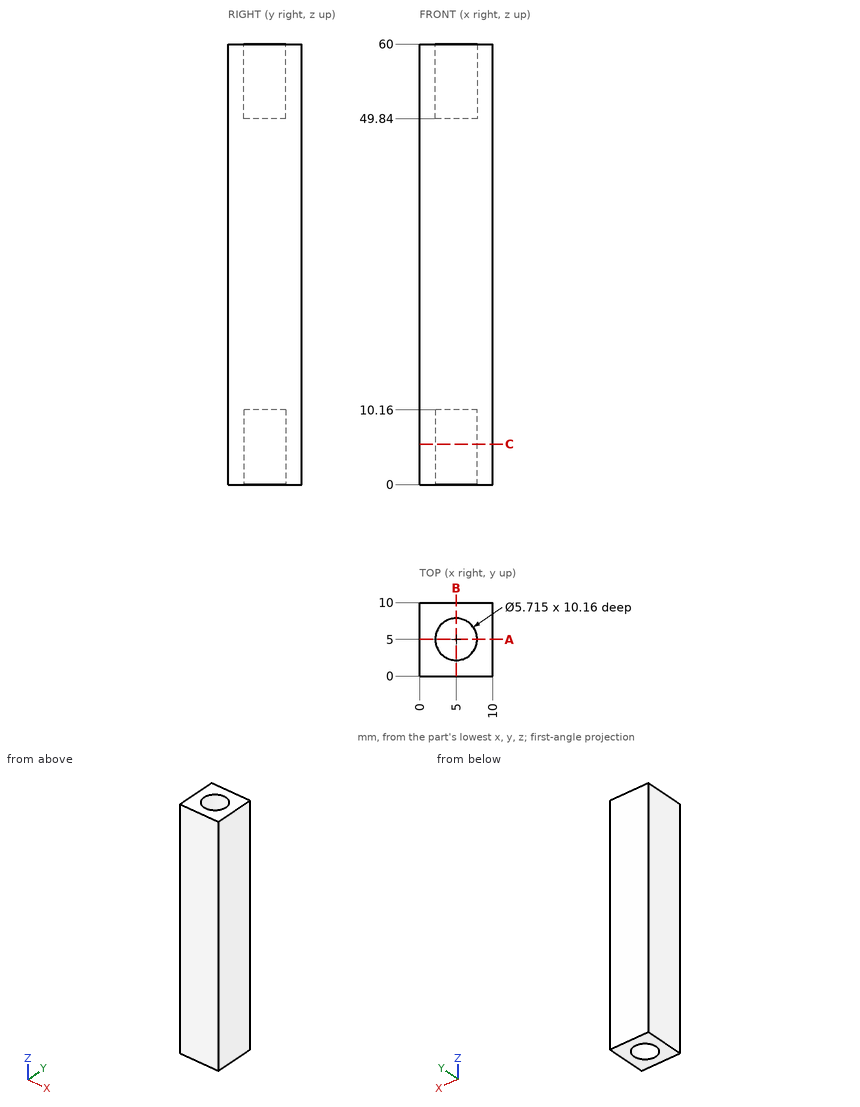
The drawing under review shows one solid part. Ordinate dimensions are in mm from its lowest x, y, z. Coordinates: 2 decimals unless noted, no trailing zeros. Order: outer loops, then holes, each group sorted by start corner. A loop starts at its lowest first (then second) coordinate and runs counter-clockwise, first axis right, second up. Notation, with made-up numbers: (-15.5, -24.5) -> (29.5, -24.5) arc R13 cw to (29.5, -19.5) -> close; hole circle Ø11 at (-11.75, 85). An arc over 180 degrees is marked (long way). Answer in a Markdown table with one row per item. Add a question column.
Item 1: To check wall thickness, follow probe 1 along Y at (x, z) = (5, 54); probe 2 along Z at (x, y) = (5, 5); probe 3 along X at (y, z) = (6, 51.5). State the ranges of each line that lie inside material, in increasing order.
Item 2: We need section A-A on y = 5. Write out the cut boundary in (x, z).
Item 3: We need section C-C on z = 5.5. Write out the cut boundary in (x, y) (1 decimal), plus the area to 3 significant figures.
Final values:
| question | item | result |
|---|---|---|
| 1 | probe 1 | y = 0 to 2.14, 7.86 to 10 |
| 1 | probe 2 | z = 10.16 to 49.84 |
| 1 | probe 3 | x = 0 to 2.32, 7.68 to 10 |
| 2 | outline | (0, 0) -> (2.14, 0) -> (2.14, 10.16) -> (7.86, 10.16) -> (7.86, 0) -> (10, 0) -> (10, 60) -> (7.86, 60) -> (7.86, 49.84) -> (2.14, 49.84) -> (2.14, 60) -> (0, 60) -> close |
| 3 | outline | (0, 0) -> (10, 0) -> (10, 10) -> (0, 10) -> close; hole circle Ø5.7 at (5, 5) |
| 3 | area | 74.3 mm2 |
